Design review of the part built by this model. Coordinates are the model's own, in mm. Face numbers are marked on the shaded views. A direction names the side the tool comes from. Coordinates: 2 decimals unless noted, no trailing zeros. Loops run counter-clockwise (first coordinate to the right, second up) from the corner with the lowest first, then second, coordinate; pieces in that order, holes last. Notation, with made-up numbers: (74, 56) - (102, 56) arc R25 cw to (102, 71) - close; hole circle Ø11 at (73, 88). An arc over 180 degrees is marked (long way). Answer in a Markdown table with one row per item. Add a question column.
(1) We need section A-A, the plane x = 0. Write out the cut boundary in (y, z), plus the area to 3 significant figures.
(2) We need section C-C, the plane y = 21. Write out the cut boundary in (x, z), plus the area to 3 significant figures.
(3) For the marked faces 1, 2, 3, 4 and 5, list the 3-axis set-ups (+Z, -Z, +X, -X, +Y, -Y) from which the entire face can be reached by the end or side of a thin tool; tool diameter is ignored.
(4) To check wall thickness, follow L1, parallel to Y at x = 1.5, z = 7.75; L2, parallel to Y at x = 0, z = 2.75; L3, parallel to Z at x = 4.75, y = 3. State the ranges of each line that lie inside material, in increasing order. Write a range as [from, to].
(5) We need section B-B, the plane y = -2.5. Write out the cut boundary in (x, z) (3 decimals), plus the area to 3 significant figures.
(6) Clearance check with flat-ended pins moving along their axes: pin 1 (3 mm diameter, centred on y = -0.5, z = 7.5, fed in from +X); pin 2 (4 mm diameter, centred on y = 2.5, z = 1.5, fed in from -X); pin 3 (2 mm diameter, centred on x = -5, z = 2, fed in from -Y). State where each tip first meets the part, or that it passes through.
from build123d import *

# Parameters (mm, degrees)
F0_W      = 11.91
F0_H      = 15.5
F1_DEPTH  = 9.98
F3_DEPTH  = 25.4
F4_R      = 2.5
F5_DEPTH  = 1.25
F6_W      = 11.91
F6_H      = 9.98
F7_DEPTH  = 9
F8_R      = 2
F9_DEPTH  = 0.81
F10_R     = 1.5
F11_DEPTH = 9.55
F12_R     = 0.5


with BuildPart() as f1:
    # F0 (on Top) → F1 (new body)
    with BuildSketch(Plane.XY):
        Rectangle(F0_W, F0_H)
    extrude(amount=F1_DEPTH)

    # F2 (on face) → F3 (cut)
    with BuildSketch(Plane.XZ.offset(7.75)):
        with BuildLine():
            ThreePointArc((-3.955, 0), (-5.955, 4.99), (-3.955, 9.98))
            Line((-3.955, 9.98), (-7.13, 9.98))
            Line((-7.13, 9.98), (-7.13, 0))
            Line((-7.13, 0), (-3.955, 0))
        make_face()
        with BuildLine():
            Line((7.13, 9.98), (3.955, 9.98))
            ThreePointArc((3.955, 9.98), (5.955, 4.99), (3.955, 0))
            Line((3.955, 0), (7.13, 0))
            Line((7.13, 0), (7.13, 9.98))
        make_face()
    extrude(amount=-F3_DEPTH, mode=Mode.SUBTRACT)

    # F4 (on face) → F5 (join)
    with BuildSketch(Plane.XZ.offset(7.75)):
        with Locations((0, 4.99)):
            Circle(F4_R)
    extrude(amount=F5_DEPTH)

    # F6 (on face) → F7 (join)
    with BuildSketch(Plane(origin=(0, 7.75, 0), x_dir=(-1, 0, 0), z_dir=(0, 1, 0))):
        with Locations((0, 4.99)):
            Rectangle(F6_W, F6_H)
    extrude(amount=F7_DEPTH)

    # F8 (on face) → F9 (join)
    with BuildSketch(Plane(origin=(0, 16.75, 0), x_dir=(-1, 0, 0), z_dir=(0, 1, 0))):
        with Locations((0, 4.99)):
            Circle(F8_R)
    extrude(amount=F9_DEPTH)

    # F10 (on face) → F11 (join)
    with BuildSketch(Plane(origin=(0, 17.56, 0), x_dir=(-1, 0, 0), z_dir=(0, 1, 0))):
        with Locations((0, 4.99)):
            Circle(F10_R)
    extrude(amount=F11_DEPTH)

    # F12
    f12_edges = [f1.edges().sort_by_distance(p)[0] for p in [
        (5.955, 12.25, 9.98),
        (-5.955, 12.25, 9.98),
        (5.955, 12.25, 0),
        (-5.955, 12.25, 0),
    ]]
    fillet(f12_edges, radius=F12_R)


solid = f1.part
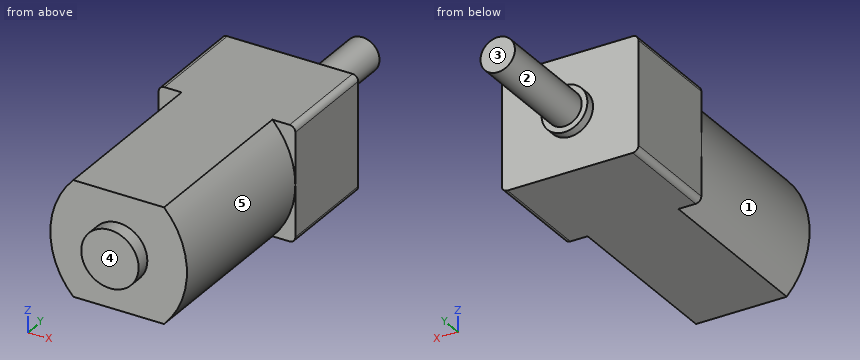
Responses:
| question | item | result |
|---|---|---|
| 1 | outline | (-9, 2.49) - (-7.75, 2.49) - (-7.75, 0) - (16.75, 0) - (16.75, 2.99) - (17.56, 2.99) - (17.56, 3.49) - (27.11, 3.49) - (27.11, 6.49) - (17.56, 6.49) - (17.56, 6.99) - (16.75, 6.99) - (16.75, 9.98) - (-7.75, 9.98) - (-7.75, 7.49) - (-9, 7.49) - close |
| 1 | area | 283 mm2 |
| 2 | outline | circle Ø3 at (0, 4.99) |
| 2 | area | 7.07 mm2 |
| 3 | face 1 | -X, -Y |
| 3 | face 2 | +Y |
| 3 | face 3 | +Z, -Z, +X, -X, +Y |
| 3 | face 4 | +Z, -Z, +X, -X, -Y |
| 3 | face 5 | +X, -Y |
| 4 | L1 | y = [-7.75, 16.75] |
| 4 | L2 | y = [-9, 16.75] |
| 4 | L3 | z = [0.99, 8.99] |
| 5 | outline | (-3.955, 0) - (3.955, 0) arc R7.225 ccw to (3.955, 9.98) - (-3.955, 9.98) arc R7.225 ccw to start |
| 5 | area | 106 mm2 |
| 6 | pin 1 | stops at x = 5.88 |
| 6 | pin 2 | stops at x = -5.8 |
| 6 | pin 3 | stops at y = -7.75 |
